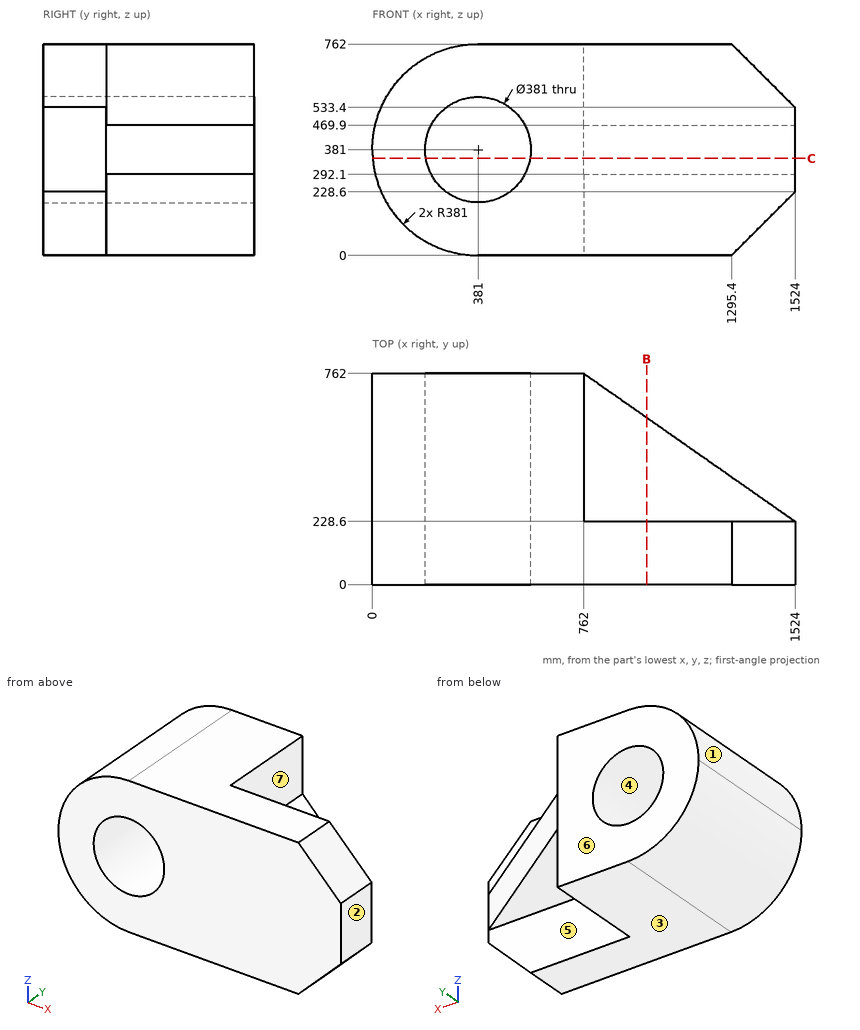
Study the drawing (mm; zero at the part's minimum x, y, z) and answer. A direction names the side the tool comes from. Coordinates: 2 decimals unless noted, no trailing zeros. Write each loop counter-clockwise with the first axis right and the second up, starting at its lowest first coordinate (ties: lowest second). Pieces come first, ordered by that corner, then holes. Notation, with made-up numbers: (76.25, 84) - (104.25, 84) arc R9 cw to (104.25, 89) - close; hole circle Ø3 at (6, 19.5). An arc over 180 degrees is marked (long way). Return JSON: item names as keys, results as strings. Group by question number.
1. A cutting plane is placed at C-C, the plane z = 349.5. Determine the outline of the cut face in (x, y), plus the area to 3 significant figures.
2. Straight lines are drawn through the part: L1, parallel to X at y = 179, z = 381; L2, parallel to Y at x = 839.5, z = 645.5; L3, parallel to Z at x = 878, y = 532. For each, find the intervals that lie inside material, in ascending order.
3. A cutting plane is placed at B-B, the plane x = 989. Determine the outline of the cut face in (y, z), plus the area to 3 significant figures.
4. Which of the six approach directions +Z, -Z, +X, -X, +Y, -Y give full straight-line access (tool end or side, diameter ignored) to the marked faces 5, 6 and 7?
5. Determine the mould class of the marked faces 1, 2, 3 and 4 for opening direction X: released by +X, released by -X, zero draft, split by the parting line, or undercut.
6. Given pin 1 (1 mm diameter, centred on y = 504, z = 489, fed in from +X); pin 2 (12 mm diameter, centred on y = 118.5, z = 673.5, fed in from -X) (1 decimal); pin 3 (10 mm diameter, centred on y = 184, z = 182.5, fed in from -X), each flat-ended and moving along its own axis, determine where each tip first touches the part or whether it passes through.
Ans:
{
 "1": {"outline": "(1.3, 0) - (193.12, 0) - (193.12, 762) - (1.3, 762) - close; (568.88, 0) - (1524, 0) - (1524, 228.6) - (762, 762) - (568.88, 762) - close", "area": "671,000 mm²"},
 "2": {"L1": "0 to 190.5, 571.5 to 1524", "L2": "0 to 228.6", "L3": "292.1 to 469.9"},
 "3": {"outline": "(0, 0) - (228.6, 0) - (228.6, 292.1) - (603.1, 292.1) - (603.1, 469.9) - (228.6, 469.9) - (228.6, 762) - (0, 762) - close", "area": "241,000 mm²"},
 "4": {"face 5": "-Z, +X, +Y", "face 6": "+Z, -Z, +X, -X, +Y", "face 7": "+Z, +X, +Y"},
 "5": {"face 1": "released by -X", "face 2": "released by +X", "face 3": "zero draft", "face 4": "undercut"},
 "6": {"pin 1": "x = 762", "pin 2": "x = 129.8", "pin 3": "x = 52.79"}
}
